Model file for the job. Use its own axes, mm. Face numbers are marked on the shaded views. Give positions to 0.01 mm unless a question says otherwise; leave off trailing zeros. Order: outer loops, then holes, each group sorted by start corner. A loop starts at its lowest first (then second) coordinate and runs counter-clockwise, first axis right, second up. Notation, with made-up numbers: (-27.5, 86.5) - (-20.5, 86.5) arc R35 cw to (-20.5, 124.5) - close; hole circle Ø7 at (35.25, 59.25). An arc over 180 degrees is marked (long way). Return JSON: item names as keys, results as strings. Group by question number.
from build123d import *

# Parameters (mm, degrees)
SKETCH16_R               = 38.448520448
BOSS_EXTRUDE3_DEPTH      = 150
SKETCH17_R               = 26.04625397
CUT_EXTRUDE2_DEPTH       = 1
CUT_EXTRUDE2_DEPTH_BACK  = 151
SKETCH18_R               = 18.685585603
CUT_EXTRUDE3_DEPTH       = 39.448520448
CUT_EXTRUDE3_DEPTH_BACK  = 1
SKETCH19_W               = 53.228745634
SKETCH19_H               = 53.407658992
BOSS_EXTRUDE4_DEPTH      = 45
BOSS_EXTRUDE4_DEPTH_BACK = 1
SKETCH20_R               = 22.488274744
CUT_EXTRUDE4_DEPTH       = 46
CUT_EXTRUDE4_DEPTH_BACK  = 1
SKETCH21_W               = 53.228745634
SKETCH21_H               = 53.043515862
BOSS_EXTRUDE5_DEPTH      = 45
SKETCH22_R               = 6.364118175
CUT_EXTRUDE5_DEPTH       = 55
CUT_EXTRUDE5_DEPTH_BACK  = 1


with BuildPart() as part:
    # Sketch16 → Boss-Extrude3 (new body)
    with BuildSketch(Plane.XY):
        Circle(SKETCH16_R)
    extrude(amount=BOSS_EXTRUDE3_DEPTH)

    # Sketch17 → Cut-Extrude2 (cut, two sides)
    with BuildSketch(Plane.XY.offset(150)) as cut_extrude2_sk:
        Circle(SKETCH17_R)
    extrude(amount=CUT_EXTRUDE2_DEPTH, mode=Mode.SUBTRACT)
    extrude(cut_extrude2_sk.sketch, amount=-CUT_EXTRUDE2_DEPTH_BACK, mode=Mode.SUBTRACT)

    # Sketch18 → Cut-Extrude3 (cut, two sides)
    with BuildSketch(Plane(origin=(0, 0, 0), x_dir=(1, 0, 0), z_dir=(0, 1, 0))) as cut_extrude3_sk:
        with Locations((0, -71.055116097)):
            Circle(SKETCH18_R)
    extrude(amount=CUT_EXTRUDE3_DEPTH, mode=Mode.SUBTRACT)
    extrude(cut_extrude3_sk.sketch, amount=-CUT_EXTRUDE3_DEPTH_BACK, mode=Mode.SUBTRACT)

    # Sketch19 → Boss-Extrude4 (add, two sides)
    with BuildSketch(Plane(origin=(0, 0, 0), x_dir=(1, 0, 0), z_dir=(0, 1, 0))) as boss_extrude4_sk:
        with Locations((0, -71.055116097)):
            Rectangle(SKETCH19_W, SKETCH19_H)
    extrude(amount=BOSS_EXTRUDE4_DEPTH)
    extrude(boss_extrude4_sk.sketch, amount=-BOSS_EXTRUDE4_DEPTH_BACK)

    # Sketch20 → Cut-Extrude4 (cut, two sides)
    with BuildSketch(Plane(origin=(0, 0, 0), x_dir=(1, 0, 0), z_dir=(0, 1, 0))) as cut_extrude4_sk:
        with Locations((0, -71.055116097)):
            Circle(SKETCH20_R)
    extrude(amount=CUT_EXTRUDE4_DEPTH, mode=Mode.SUBTRACT)
    extrude(cut_extrude4_sk.sketch, amount=-CUT_EXTRUDE4_DEPTH_BACK, mode=Mode.SUBTRACT)

    # Sketch21 → Boss-Extrude5 (add)
    with BuildSketch(Plane(origin=(0, 0, 0), x_dir=(1, 0, 0), z_dir=(0, 1, 0))):
        with Locations((0, -71.237187662)):
            Rectangle(SKETCH21_W, SKETCH21_H)
    extrude(amount=BOSS_EXTRUDE5_DEPTH)

    # Sketch22 → Cut-Extrude5 (cut, two sides)
    with BuildSketch(Plane(origin=(0, 0, 0), x_dir=(1, 0, 0), z_dir=(0, 1, 0))) as cut_extrude5_sk:
        with Locations((-0.905733708, -73.105080143)):
            Circle(SKETCH22_R)
    extrude(amount=CUT_EXTRUDE5_DEPTH, mode=Mode.SUBTRACT)
    extrude(cut_extrude5_sk.sketch, amount=-CUT_EXTRUDE5_DEPTH_BACK, mode=Mode.SUBTRACT)


solid = part.part
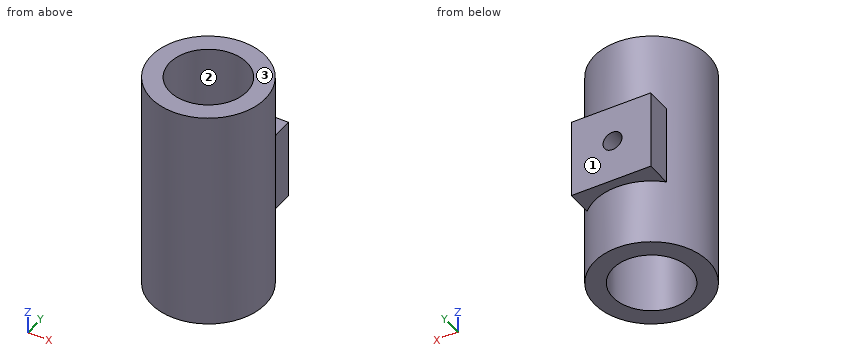
(1) Pull direction Y, two halves, no side cores. Call the marked faces 1, 2 and 3: released by +Y, released by -Y, zero draft, split by the parting line, or undercut.
(2) Drill centre lines: L1, parallel to Y at x = 0, z = 110; L2, parallel to Z at x = -1, y = 40; L3, parallel to Z at x = 8.5, y = 3. Where is each one in solid material? Low to high.
(3) Slice it at C-C (x = -15). Give the cut face in (y, z).
(4) Slice it at B-B (y = 12). Give the cut face in (x, z).
(5) Slice it at A-A (x = 0). Give the cut face in (y, z).
(6) Drop flat-ended pins along their axis: pin 1 Ø13.5 at (x, z) = (4, 82) entering from -Y; pin 2 Ø5 at (y, z) = (-26, 98.5) entering from +X; pin 3 Ø8.5 at (y, z) = (32.5, 77.5) entering from -X; pin 4 Ø19 at (x, y) = (11.5, 40) entering from +Z. Give the stop position or say it passes through.
(7) Slice it at D-D (z = 34.5). Give the cut face in (x, y).
Result set:
{
 "1": {"face 1": "released by +Y", "face 2": "undercut", "face 3": "zero draft"},
 "2": {"L1": "y = -38.45 to -26.05, 26.05 to 38.45", "L2": "z = 44.35 to 66.74, 79.47 to 97.76", "L3": "z = 44.35 to 97.76"},
 "3": {"outline": "(-35.4, 0) - (-21.29, 0) - (-21.29, 150) - (-35.4, 150) - close; (-1, 44.35) - (21.29, 44.35) - (21.29, 0) - (35.4, 0) - (35.4, 44.35) - (45, 44.35) - (45, 97.76) - (35.4, 97.76) - (35.4, 150) - (21.29, 150) - (21.29, 97.76) - (-1, 97.76) - (-1, 87.81) - (0, 87.81) - (0, 54.3) - (-1, 54.3) - close"},
 "4": {"outline": "(-36.53, 0) - (-23.12, 0) - (-23.12, 44.35) - (23.12, 44.35) - (23.12, 0) - (36.53, 0) - (36.53, 150) - (23.12, 150) - (23.12, 97.76) - (-23.12, 97.76) - (-23.12, 150) - (-36.53, 150) - close; hole circle Ø12.73 at (-0.91, 73.11)"},
 "5": {"outline": "(-38.45, 0) - (-26.05, 0) - (-26.05, 150) - (-38.45, 150) - close; (-1, 44.35) - (26.05, 44.35) - (26.05, 0) - (38.45, 0) - (38.45, 44.35) - (45, 44.35) - (45, 66.81) - (0, 66.81) - (0, 48.57) - (-1, 48.57) - close; (-1, 93.54) - (0, 93.54) - (0, 79.4) - (45, 79.4) - (45, 97.76) - (38.45, 97.76) - (38.45, 150) - (26.05, 150) - (26.05, 97.76) - (-1, 97.76) - close"},
 "6": {"pin 1": "stops at y = -38.45", "pin 2": "stops at x = 30.43", "pin 3": "stops at x = -26.61", "pin 4": "stops at z = 150"},
 "7": {"outline": "circle Ø76.9 at (0, 0); hole circle Ø52.09 at (0, 0)"}
}
